Solid Edge part; units mm, degrees
sketch "Sketch1" plane through (0, 0, 0) normal (0, 0, 1) x (1, 0, 0)
  circle A0 centre (0, 0) radius 2.413
extrude "Protrusion1" add sketch "Sketch1" along normal blind 38.1
chamfer "Chamfer1" distance 0.3619 angle 45 2 edges at (-2.413, 0, 0) (-2.413, 0, 38.1)
sketch "Sketch2" plane through (0, 0, 38.1) normal (0, 0, 1) x (1, 0, 0)
  line L0 (-0.6878, 1.1913) -> (0.6878, 1.1913)
  line L1 (1.3755, 0) -> (0.6878, 1.1913)
  line L2 (0.6878, -1.1913) -> (1.3755, 0)
  line L3 (-0.6878, -1.1913) -> (0.6878, -1.1913)
  line L4 (-1.3755, 0) -> (-0.6878, -1.1913)
  line L5 (-0.6878, 1.1913) -> (-1.3755, 0)
extrude "Cutout1" cut sketch "Sketch2" against normal blind 19.05
properties part number "24101312"
Design review of the part built by this model. Coordinates are the model's own, in mm. A direction names the side the tool comes from. Round coordinates to 2 decimals unless told otherwise and drop trailing zeros. Write each loop counter-clockwise with the first axis right and the second up, starting at its lowest first coordinate (ties: lowest second). Pieces come first, ordered by that corner, then holes. Notation, with made-up numbers: (6.25, 9) - (51.25, 9) arc R35 cw to (51.25, 48) - close; hole circle Ø1 at (-16.75, 60). An arc over 180 degrees is marked (long way). Use a Markdown table: item, result. Add a question column.
1. Clearance check with a flat-ended pin moving along its axis: pin 1 (1.2 mm diameter, centred on x = 0.5, y = 0, fed in from +Z). State where the tip first meets the part, or that it passes through.
2. For faces 1 (the face through (-1.03, 0.6, 28.71)), 2 (the face through (1, -1, 38.1)), list the 3-axis set-ups (+Z, -Z, +X, -X, +Y, -Y) from which the entire face can be reached by the end or side of a thin tool; tool diameter is ignored.
3. Mouldability with a two-part tool opening along X and no side actions: class faces 3 (the face through (-1.915, 1.468, 18.788)), 4 (the face through (1.036, 0.587, 28.708)), 5 (the face through (0, 0, 0)) as +X half, -X half, draft (parallel to the pull), parting line (faces both ways), or undercut.
4. We need section B-B (x = 0). State the section outline as (y, z) points, then the cut area to 3 significant figures.
5. We need section C-C (z = 14). State the section outline as (x, y) points.
6. Wall thickness on probe 1 along Y at (x, z) = (0.1, 23); probe 2 along Y at (x, z) = (0.2, 15); probe 3 along Z at (x, y) = (0.3, -1): over which ranges is each line inside the solid? List them lowest first.
7. We need section A-A (z = 24.5). State the section outline as (x, y) points, then the cut area to 3 significant figures.
Output:
| question | item | result |
|---|---|---|
| 1 | pin 1 | stops at z = 19.05 |
| 2 | face 1 | +Z |
| 2 | face 2 | +Z, +X, -X, +Y, -Y |
| 3 | face 3 | parting line |
| 3 | face 4 | undercut |
| 3 | face 5 | draft |
| 4 | outline | (-2.41, 0.36) - (-2.05, 0) - (2.05, 0) - (2.41, 0.36) - (2.41, 37.74) - (2.05, 38.1) - (1.19, 38.1) - (1.19, 19.05) - (-1.19, 19.05) - (-1.19, 38.1) - (-2.05, 38.1) - (-2.41, 37.74) - close |
| 4 | area | 138 mm2 |
| 5 | outline | circle Ø4.83 at (0, 0) |
| 6 | probe 1 | y = -2.41 to -1.19, 1.19 to 2.41 |
| 6 | probe 2 | y = -2.4 to 2.4 |
| 6 | probe 3 | z = 0 to 19.05 |
| 7 | outline | circle Ø4.83 at (0, 0); hole (-1.38, 0) - (-0.69, -1.19) - (0.69, -1.19) - (1.38, 0) - (0.69, 1.19) - (-0.69, 1.19) - close |
| 7 | area | 13.4 mm2 |
